from build123d import *

# Parameters (mm, degrees)
F1_DEPTH = 3.175
F2_W     = 44.45
F2_H     = 19.05
F3_DEPTH = 6.35


with BuildPart() as f1:
    # F0 (on Front) → F1 (new body, symmetric)
    with BuildSketch(Plane.XZ):
        with BuildLine():
            Line((-22.225, 69.85), (-22.225, 0))
            Line((-22.225, 0), (22.225, 0))
            Line((22.225, 0), (22.225, 69.85))
            ThreePointArc((22.225, 69.85), (0, 56.746722), (-22.225, 69.85))
        make_face()
    extrude(amount=F1_DEPTH, both=True)

    # F2 (on face) → F3 (join)
    with BuildSketch(Plane(origin=(0, 0, 0), x_dir=(1, 0, 0), z_dir=(0, 0, -1))):
        with Locations((0, -12.7)):
            Rectangle(F2_W, F2_H)
    extrude(amount=-F3_DEPTH)


solid = f1.part
Check sheet for the modelled part. Datum: model origin and axes. Units: mm. A direction names the side the tool comes from. Round coordinates to 2 decimals unless told otherwise and drop trailing zeros. Order: outer loops, then holes, each group sorted by start corner. A loop starts at its lowest first (then second) coordinate and runs counter-clockwise, first axis right, second up.
Q1. Depth check by flat-ended pin: P1, Ø3, axis at x = -9.5, z = 11.5, coming from the +Y side (3 decimals); P2, Ø4, axis at x = -15.5, y = 19.5, coming from the +Z side. Enter the tip coordinate at first touch or a pass-through.
Filled sheet:
P1: stops at y = 3.175
P2: stops at z = 6.35
Q2. Cross-section at C-C, the plane y = 9.5. Enter the section's corners in (x, z) (3 decimals).
Filled sheet:
outline: (-22.225, 0) - (22.225, 0) - (22.225, 6.35) - (-22.225, 6.35) - close
Q3. Set-up check for faces 4 (the face through (0, 22.225, 3)), 5 (the face through (0, 13, 6.35)): record each of +Z, -Z, +X, -X, +Y, -Y from which the full face is reachable in a straight line by a thin tool's end or side.
Filled sheet:
face 4: +Z, -Z, +X, -X, +Y
face 5: +Z, +X, -X, +Y
Q4. Cross-section at A-A, the plane z = 61. Enter the section's corners in (x, y) (3 decimals), plus the area to 3 significant figures.
Filled sheet:
outline: (-22.225, -3.175) - (-14.07, -3.175) - (-14.07, 3.175) - (-22.225, 3.175) - close; (14.07, -3.175) - (22.225, -3.175) - (22.225, 3.175) - (14.07, 3.175) - close
area: 104 mm2
Q5. Scan lines: L1, parallel to Y at x = 4, z = 9.5 (3 decimals); L2, parallel to X at y = 2.75, z = 60.5 (3 decimals); L3, parallel to Z at x = -11.5, y = 5. Record each from-to range of solid material in increasing order.
Filled sheet:
L1: y = -3.175 to 3.175
L2: x = -22.225 to -13.288, 13.288 to 22.225
L3: z = 0 to 6.35
Q6. Cross-section at D-D, the plane z = 10. Enter the section's corners in (x, y) (3 decimals), plus the area to 3 significant figures.
Filled sheet:
outline: (-22.225, -3.175) - (22.225, -3.175) - (22.225, 3.175) - (-22.225, 3.175) - close
area: 282 mm2
Q7. Draft check along X on faces 1 (the face through (-22.225, 2, 27)), 2 (the face through (0.38, -0.04, 56.75)), 3 (the face through (0, 9, 0)). Enter one of: pulls with the +X half, pulls with the -X half, needs draft (parallel to the pull), parting line crosses it, or undercut.
Filled sheet:
face 1: pulls with the -X half
face 2: undercut
face 3: needs draft
Q8. Cross-section at B-B, the plane x = -10. Enter the section's corners in (y, z) (3 decimals).
Filled sheet:
outline: (-3.175, 0) - (22.225, 0) - (22.225, 6.35) - (3.175, 6.35) - (3.175, 58.798) - (-3.175, 58.798) - close
